The model under review builds one solid part; all positions refer to its coordinate system, in mm. A direction names the side the tool comes from. Round coordinates to 2 decimals unless told otherwise and drop trailing zeros. Write each loop counter-clockwise with the first axis right and the second up, starting at its lowest first coordinate (ties: lowest second). Pieces come first, ordered by that corner, then holes. Notation, with made-up numbers: (19.5, 37) - (29.5, 37) arc R20 ccw to (29.5, 75) - close; hole circle Ø8 at (29.25, 89). An arc over 180 degrees is marked (long way). One line per question, with ' | ' between items. Start each with the question number.
```python
from build123d import *

# Parameters (mm, degrees)
SKETCH3_R           = 9.9
BOSS_EXTRUDE1_DEPTH = 75
SKETCH7_W           = 3.24
SKETCH7_H           = 3.24
CUT_EXTRUDE8_DEPTH  = 10.2
CUT_EXTRUDE9_DEPTH  = 4.2
SKETCH7_7_R         = 4.7
SKETCH7_7_R_2       = 2.7
CUT_EXTRUDE10_DEPTH = 2.2
BOSS_EXTRUDE3_START = 10
BOSS_EXTRUDE3_DEPTH = 10
CUT_EXTRUDE11_DEPTH = 10


with BuildPart() as part:
    # Sketch3 → Boss-Extrude1 (new body)
    with BuildSketch(Plane(origin=(0, 0, 0), x_dir=(1, 0, 0), z_dir=(0, 1, 0))):
        with Locations(Location((0, 0, 0), (0, 0, 270))):
            Circle(SKETCH3_R)
    extrude(amount=-BOSS_EXTRUDE1_DEPTH)

    # Sketch7 → Cut-Extrude8 (cut)
    with BuildSketch(Plane(origin=(0, -75, 0), x_dir=(-1, 0, 0), z_dir=(0, -1, 0))):
        with BuildLine():
            Line((1.62, -1.62), (-1.62, -1.62))
            Line((-1.62, -1.62), (-1.62, -2.16))
            ThreePointArc((-1.62, -2.16), (0, -2.7), (1.62, -2.16))
            Line((1.62, -2.16), (1.62, -1.62))
        make_face()
        Rectangle(SKETCH7_W, SKETCH7_H)
        with BuildLine():
            Line((-1.62, 2.16), (-1.62, 1.62))
            Line((-1.62, 1.62), (1.62, 1.62))
            Line((1.62, 1.62), (1.62, 2.16))
            ThreePointArc((1.62, 2.16), (0, 2.7), (-1.62, 2.16))
        make_face()
    extrude(amount=-CUT_EXTRUDE8_DEPTH, mode=Mode.SUBTRACT)

    # Sketch7_6 → Cut-Extrude9 (cut)
    with BuildSketch(Plane(origin=(0, -75, 0), x_dir=(-1, 0, 0), z_dir=(0, -1, 0))):
        with BuildLine():
            Line((1.62, 2.16), (1.62, 1.62))
            Line((1.62, 1.62), (2.16, 1.62))
            ThreePointArc((2.16, 1.62), (1.909188309, 1.909188309), (1.62, 2.16))
        make_face()
        with BuildLine():
            Line((2.16, 1.62), (1.62, 1.62))
            Line((1.62, 1.62), (1.62, -1.62))
            Line((1.62, -1.62), (2.16, -1.62))
            ThreePointArc((2.16, -1.62), (2.561444905, -0.853814968), (2.7, 0))
            ThreePointArc((2.7, 0), (2.561444905, 0.853814968), (2.16, 1.62))
        make_face()
        with BuildLine():
            Line((2.16, -1.62), (1.62, -1.62))
            Line((1.62, -1.62), (1.62, -2.16))
            ThreePointArc((1.62, -2.16), (1.909188309, -1.909188309), (2.16, -1.62))
        make_face()
        with BuildLine():
            Line((-1.62, -1.62), (-2.16, -1.62))
            ThreePointArc((-2.16, -1.62), (-1.909188309, -1.909188309), (-1.62, -2.16))
            Line((-1.62, -2.16), (-1.62, -1.62))
        make_face()
        with BuildLine():
            Line((-1.62, 1.62), (-2.16, 1.62))
            ThreePointArc((-2.16, 1.62), (-2.7, 0), (-2.16, -1.62))
            Line((-2.16, -1.62), (-1.62, -1.62))
            Line((-1.62, -1.62), (-1.62, 1.62))
        make_face()
        with BuildLine():
            ThreePointArc((-1.62, 2.16), (-1.909188309, 1.909188309), (-2.16, 1.62))
            Line((-2.16, 1.62), (-1.62, 1.62))
            Line((-1.62, 1.62), (-1.62, 2.16))
        make_face()
    extrude(amount=-CUT_EXTRUDE9_DEPTH, mode=Mode.SUBTRACT)

    # Sketch7_7 → Cut-Extrude10 (cut)
    with BuildSketch(Plane(origin=(0, -75, 0), x_dir=(-1, 0, 0), z_dir=(0, -1, 0))):
        with Locations(Location((0, 0, 0), (0, 0, 90))):
            Circle(SKETCH7_7_R)
        with Locations(Location((0, 0, 0), (0, 0, 90))):
            Circle(SKETCH7_7_R_2, mode=Mode.SUBTRACT)
    extrude(amount=-CUT_EXTRUDE10_DEPTH, mode=Mode.SUBTRACT)

    # Sketch5 → Boss-Extrude3 (add)
    with BuildSketch(Plane(origin=(0, 0, 0), x_dir=(1, 0, 0), z_dir=(0, 1, 0)).offset(BOSS_EXTRUDE3_START)):
        with BuildLine():
            Line((-2, 9.695875412), (-2, 2))
            Line((-2, 2), (-9.695875412, 2))
            ThreePointArc((-9.695875412, 2), (-9.9, 0), (-9.695875412, -2))
            Line((-9.695875412, -2), (-2, -2))
            Line((-2, -2), (-2, -9.695875412))
            ThreePointArc((-2, -9.695875412), (0, -9.9), (2, -9.695875412))
            Line((2, -9.695875412), (2, -2))
            Line((2, -2), (9.695875412, -2))
            ThreePointArc((9.695875412, -2), (9.848836646, -1.005194863), (9.9, 0))
            ThreePointArc((9.9, 0), (9.848836646, 1.005194863), (9.695875412, 2))
            Line((9.695875412, 2), (2, 2))
            Line((2, 2), (2, 9.695875412))
            ThreePointArc((2, 9.695875412), (0, 9.9), (-2, 9.695875412))
        make_face()
    extrude(amount=-BOSS_EXTRUDE3_DEPTH)

    # Sketch11 → Cut-Extrude11 (cut)
    with BuildSketch(Plane(origin=(0, 10, 0), x_dir=(1, 0, 0), z_dir=(0, 1, 0))):
        with BuildLine():
            Line((-1.9, 1.9), (-1.9, 9.614052215))
            ThreePointArc((-1.9, 9.614052215), (-1.950026427, 9.604030244), (-2, 9.593747964))
            Line((-2, 9.593747964), (-2, 2))
            Line((-2, 2), (-9.593747964, 2))
            ThreePointArc((-9.593747964, 2), (-9.604030244, 1.950026427), (-9.614052215, 1.9))
            Line((-9.614052215, 1.9), (-1.9, 1.9))
        make_face()
        with BuildLine():
            Line((-1.9, 9.614052215), (-1.9, 9.715966241))
            ThreePointArc((-1.9, 9.715966241), (-1.950025874, 9.706049613), (-2, 9.695875412))
            Line((-2, 9.695875412), (-2, 9.593747964))
            ThreePointArc((-2, 9.593747964), (-1.950026427, 9.604030244), (-1.9, 9.614052215))
        make_face()
        with BuildLine():
            ThreePointArc((1.9, 9.715966241), (0, 9.9), (-1.9, 9.715966241))
            Line((-1.9, 9.715966241), (-1.9, 9.614052215))
            ThreePointArc((-1.9, 9.614052215), (0, 9.8), (1.9, 9.614052215))
            Line((1.9, 9.614052215), (1.9, 9.715966241))
        make_face()
        with BuildLine():
            ThreePointArc((2, 9.695875412), (1.950025874, 9.706049613), (1.9, 9.715966241))
            Line((1.9, 9.715966241), (1.9, 9.614052215))
            ThreePointArc((1.9, 9.614052215), (1.950026427, 9.604030244), (2, 9.593747964))
            Line((2, 9.593747964), (2, 9.695875412))
        make_face()
        with BuildLine():
            ThreePointArc((2, 9.593747964), (1.950026427, 9.604030244), (1.9, 9.614052215))
            Line((1.9, 9.614052215), (1.9, 1.9))
            Line((1.9, 1.9), (9.614052215, 1.9))
            ThreePointArc((9.614052215, 1.9), (9.604030244, 1.950026427), (9.593747964, 2))
            Line((9.593747964, 2), (2, 2))
            Line((2, 2), (2, 9.593747964))
        make_face()
        with BuildLine():
            ThreePointArc((9.715966241, 1.9), (9.706049613, 1.950025874), (9.695875412, 2))
            Line((9.695875412, 2), (9.593747964, 2))
            ThreePointArc((9.593747964, 2), (9.604030244, 1.950026427), (9.614052215, 1.9))
            Line((9.614052215, 1.9), (9.715966241, 1.9))
        make_face()
        with BuildLine():
            Line((9.715966241, 1.9), (9.614052215, 1.9))
            ThreePointArc((9.614052215, 1.9), (9.753402271, 0.954538708), (9.8, 0))
            ThreePointArc((9.8, 0), (9.753402271, -0.954538708), (9.614052215, -1.9))
            Line((9.614052215, -1.9), (9.715966241, -1.9))
            ThreePointArc((9.715966241, -1.9), (9.853884153, -0.954445968), (9.9, 0))
            ThreePointArc((9.9, 0), (9.853884153, 0.954445968), (9.715966241, 1.9))
        make_face()
        with BuildLine():
            Line((9.715966241, -1.9), (9.614052215, -1.9))
            ThreePointArc((9.614052215, -1.9), (9.604030244, -1.950026427), (9.593747964, -2))
            Line((9.593747964, -2), (9.695875412, -2))
            ThreePointArc((9.695875412, -2), (9.706049613, -1.950025874), (9.715966241, -1.9))
        make_face()
        with BuildLine():
            Line((9.614052215, -1.9), (1.9, -1.9))
            Line((1.9, -1.9), (1.9, -9.614052215))
            ThreePointArc((1.9, -9.614052215), (1.950026427, -9.604030244), (2, -9.593747964))
            Line((2, -9.593747964), (2, -2))
            Line((2, -2), (9.593747964, -2))
            ThreePointArc((9.593747964, -2), (9.604030244, -1.950026427), (9.614052215, -1.9))
        make_face()
        with BuildLine():
            ThreePointArc((2, -9.593747964), (1.950026427, -9.604030244), (1.9, -9.614052215))
            Line((1.9, -9.614052215), (1.9, -9.715966241))
            ThreePointArc((1.9, -9.715966241), (1.950025874, -9.706049613), (2, -9.695875412))
            Line((2, -9.695875412), (2, -9.593747964))
        make_face()
        with BuildLine():
            ThreePointArc((1.9, -9.614052215), (0, -9.8), (-1.9, -9.614052215))
            Line((-1.9, -9.614052215), (-1.9, -9.715966241))
            ThreePointArc((-1.9, -9.715966241), (0, -9.9), (1.9, -9.715966241))
            Line((1.9, -9.715966241), (1.9, -9.614052215))
        make_face()
        with BuildLine():
            Line((-1.9, -9.715966241), (-1.9, -9.614052215))
            ThreePointArc((-1.9, -9.614052215), (-1.950026427, -9.604030244), (-2, -9.593747964))
            Line((-2, -9.593747964), (-2, -9.695875412))
            ThreePointArc((-2, -9.695875412), (-1.950025874, -9.706049613), (-1.9, -9.715966241))
        make_face()
        with BuildLine():
            Line((-1.9, -9.614052215), (-1.9, -1.9))
            Line((-1.9, -1.9), (-9.614052215, -1.9))
            ThreePointArc((-9.614052215, -1.9), (-9.604030244, -1.950026427), (-9.593747964, -2))
            Line((-9.593747964, -2), (-2, -2))
            Line((-2, -2), (-2, -9.593747964))
            ThreePointArc((-2, -9.593747964), (-1.950026427, -9.604030244), (-1.9, -9.614052215))
        make_face()
        with BuildLine():
            Line((-9.593747964, 2), (-9.695875412, 2))
            ThreePointArc((-9.695875412, 2), (-9.706049613, 1.950025874), (-9.715966241, 1.9))
            Line((-9.715966241, 1.9), (-9.614052215, 1.9))
            ThreePointArc((-9.614052215, 1.9), (-9.604030244, 1.950026427), (-9.593747964, 2))
        make_face()
        with BuildLine():
            ThreePointArc((-9.614052215, -1.9), (-9.8, 0), (-9.614052215, 1.9))
            Line((-9.614052215, 1.9), (-9.715966241, 1.9))
            ThreePointArc((-9.715966241, 1.9), (-9.9, 0), (-9.715966241, -1.9))
            Line((-9.715966241, -1.9), (-9.614052215, -1.9))
        make_face()
        with BuildLine():
            ThreePointArc((-9.593747964, -2), (-9.604030244, -1.950026427), (-9.614052215, -1.9))
            Line((-9.614052215, -1.9), (-9.715966241, -1.9))
            ThreePointArc((-9.715966241, -1.9), (-9.706049613, -1.950025874), (-9.695875412, -2))
            Line((-9.695875412, -2), (-9.593747964, -2))
        make_face()
    extrude(amount=-CUT_EXTRUDE11_DEPTH, mode=Mode.SUBTRACT)


solid = part.part
```
1. Clearance check with flat-ended pins moving along their axes: P1, Ø2, axis at y = -41.5, z = -0.5, coming from the +X side; P2, Ø2, axis at y = -24, z = 7, coming from the +X side; P3, Ø2.5, axis at y = 3, z = -5, coming from the +X side; P4, Ø6, axis at y = 3.5, z = -7, coming from the -X side. State where each tip first meets the part, or that it passes through.
2. Add section D-D, the plane x = -7. Write out the cut boundary in (y, z), then the cut area to 3 significant figures.
3. Add section B-B, the plane y = -17. Write out the cut boundary in (x, z).
4. Wall thickness on line 1 along X through (y, z) = (-73.55, 0); line 2 along Y through (x, z) = (0, -1); line 3 along Y through (x, z) = (3, 0): over which ranges is each line inside the solid? List them lowest first. Write a range as [from, to].
5. Add section A-A, the plane x = 0. Write out the cut boundary in (y, z), then the cut area to 3 significant figures.
6. Add section C-C, the plane z = -5.5. Write out the cut boundary in (x, y), then the cut area to 3 significant figures.
7. The part is to be moulded in two halves that separate along X. For faces 1 (the face through (0, 5.1, 9.8)), 2 (the face through (-2.02, -72.8, -2.02)), 3 (the face through (6, 5, -1.9)), 4 (the face through (-1.9, 5, 6)), say which applies: pulls with the +X half, pulls with the -X half, needs draft (parallel to the pull), parting line crosses it, or undercut.
8. Machinability: for faces 5 (the face through (1.412, -73.915, -4.483)), 6 (the face through (-6, 5, 1.9)), 7 (the face through (6, 5, 1.9)), 8 (the face through (-1.9, 5, -6)), which of the approach directions +Z, -Z, +X, -X, +Y, -Y give a long, thin tool a straight path to every point of the face, cutting with its end or side? Answer none if there is none.
Geometry check:
1) P1: stops at x = 9.9 | P2: stops at x = 7.87 | P3: stops at x = 1.9 | P4: stops at x = -1.9
2) outline: (-75, -7) - (0, -7) - (0, -1.9) - (10, -1.9) - (10, 1.9) - (0, 1.9) - (0, 7) - (-75, 7) - close | area: 1,090 mm2
3) outline: circle Ø19.8 at (0, 0)
4) line 1: x = [-9.9, -4.7], [4.7, 9.9] | line 2: y = [-64.8, 10] | line 3: y = [-72.8, 10]
5) outline: (-75, -9.9) - (0, -9.9) - (0, -9.8) - (10, -9.8) - (10, 9.8) - (0, 9.8) - (0, 9.9) - (-75, 9.9) - (-75, 4.7) - (-72.8, 4.7) - (-72.8, 2.7) - (-64.8, 2.7) - (-64.8, -2.7) - (-72.8, -2.7) - (-72.8, -4.7) - (-75, -4.7) - close | area: 1,620 mm2
6) outline: (-8.23, -75) - (8.23, -75) - (8.23, 0) - (1.9, 0) - (1.9, 10) - (-1.9, 10) - (-1.9, 0) - (-8.23, 0) - close | area: 1,270 mm2
7) face 1: parting line crosses it | face 2: undercut | face 3: needs draft | face 4: pulls with the -X half
8) face 5: -Y | face 6: +Z, -X, +Y | face 7: +Z, +X, +Y | face 8: -Z, -X, +Y
